Build history of the part. All positions in model axes, mm. Coordinates: 2 decimals unless noted, no trailing zeros. Order: outer loops, then holes, each group sorted by start corner. A loop starts at its lowest first (then second) coordinate and runs counter-clockwise, first axis right, second up. Notation, with made-up numbers: (87.25, 60.25) - (118.25, 60.25) arc R20 cw to (118.25, 81.25) - close; hole circle Ø3 at (47, -4.75). An arc over 180 degrees is marked (long way). Answer as CSV lines item,"result". Start each with the question number.
from build123d import *

# Parameters (mm, degrees)
SKETCH_1_W          = 160
SKETCH_1_H          = 200
EXTRUDE_2_DEPTH     = 3
SKETCH_2_R          = 1
SKETCH_2_W          = 20
SKETCH_2_H          = 40
CUT_EXTRUDE_1_DEPTH = 3
SKETCH_3_R          = 0.75
CUT_EXTRUDE_2_DEPTH = 10
SKETCH_4_R          = 1.6
CUT_EXTRUDE_3_DEPTH = 10
SKETCH_5_W          = 20
SKETCH_5_H          = 1.5
CUT_EXTRUDE_4_DEPTH = 10


with BuildPart() as part:
    # 草图1 → 凸台-拉伸2 (new body)
    with BuildSketch(Plane(origin=(0, 0, 0), x_dir=(1, 0, 0), z_dir=(0, 1, 0))):
        Rectangle(SKETCH_1_W, SKETCH_1_H)
    extrude(amount=EXTRUDE_2_DEPTH)

    # 草图2 → 切除-拉伸1 (cut)
    with BuildSketch(Plane(origin=(0, 3, 0), x_dir=(1, 0, 0), z_dir=(0, 1, 0))):
        with Locations((23, -90)):
            Circle(SKETCH_2_R)
        with Locations((13, -44)):
            Circle(SKETCH_2_R)
        with Locations((-23, -90)):
            Circle(SKETCH_2_R)
        with Locations((-23, -44)):
            Circle(SKETCH_2_R)
        with Locations((-13, -44)):
            Circle(SKETCH_2_R)
        with Locations((-13, -90)):
            Circle(SKETCH_2_R)
        with Locations((13, -90)):
            Circle(SKETCH_2_R)
        with Locations((22.939303547, -44)):
            Circle(SKETCH_2_R)
        with Locations((-18, -67)):
            Rectangle(SKETCH_2_W, SKETCH_2_H)
        with Locations((18, -67)):
            Rectangle(SKETCH_2_W, SKETCH_2_H)
    extrude(amount=-CUT_EXTRUDE_1_DEPTH, mode=Mode.SUBTRACT)

    # 草图3 → 切除-拉伸2 (cut)
    with BuildSketch(Plane(origin=(0, 3, 0), x_dir=(1, 0, 0), z_dir=(0, 1, 0))):
        with Locations((35, -10)):
            Circle(SKETCH_3_R)
        with Locations((35, 6)):
            Circle(SKETCH_3_R)
        with Locations((-1, -10)):
            Circle(SKETCH_3_R)
        with Locations((-1, 6)):
            Circle(SKETCH_3_R)
    extrude(amount=-CUT_EXTRUDE_2_DEPTH, mode=Mode.SUBTRACT)

    # 草图4 → 切除-拉伸3 (cut)
    with BuildSketch(Plane(origin=(0, 3, 0), x_dir=(1, 0, 0), z_dir=(0, 1, 0))):
        with Locations((72, 1.284440395)):
            Circle(SKETCH_4_R)
        with Locations((-72, -1.368262766)):
            Circle(SKETCH_4_R)
        with Locations((72, 92)):
            Circle(SKETCH_4_R)
        with Locations((-72, 92)):
            Circle(SKETCH_4_R)
        with Locations((-72, -92)):
            Circle(SKETCH_4_R)
        with Locations((72, -92)):
            Circle(SKETCH_4_R)
        with Locations((0, -92)):
            Circle(SKETCH_4_R)
        with Locations((0, 92)):
            Circle(SKETCH_4_R)
    extrude(amount=-CUT_EXTRUDE_3_DEPTH, mode=Mode.SUBTRACT)

    # 草图5 → 切除-拉伸4 (cut)
    with BuildSketch(Plane(origin=(0, 3, 0), x_dir=(1, 0, 0), z_dir=(0, 1, 0))):
        with Locations((-30, 77.25)):
            Rectangle(SKETCH_5_W, SKETCH_5_H)
        with Locations((-30, 30.75)):
            Rectangle(SKETCH_5_W, SKETCH_5_H)
        with Locations((15.068831665, 77.25)):
            Rectangle(SKETCH_5_W, SKETCH_5_H)
        with Locations((11.85252458, 30.75)):
            Rectangle(SKETCH_5_W, SKETCH_5_H)
    extrude(amount=-CUT_EXTRUDE_4_DEPTH, mode=Mode.SUBTRACT)


solid = part.part
(1) Probe L1, parallel to X at y = 2.3, z = 44; L2, parallel to X at y = 1.7, z = 90; L3, parallel to Z at x = 16, y = 2.8. List the from-to ranges inside material, lowest first. Write a range as [from, to].
(2) Band-saw the part on B-B on z = 80. List the corners of the cut face in (x, y), plus the area to 3 significant figures.
(3) Band-saw the part on A-A on x = -34. List the corners of the cut face in (y, z).
(4) Band-saw the part on C-C on y = 2.3. State how many separate pieces and enclosed holes the cut face has, plus the area to 3 significant figures.
Filled in:
1,L1,"x = [-80, -24], [-22, -14], [-12, 12], [14, 21.94], [23.94, 80]"
1,L2,"x = [-80, -24], [-22, -14], [-12, 12], [14, 22], [24, 80]"
1,L3,"z = [-100, -78], [-76.5, -31.5], [-30, 47], [87, 100]"
2,outline,"(-80, 0) - (-28, 0) - (-28, 3) - (-80, 3) - close; (-8, 0) - (8, 0) - (8, 3) - (-8, 3) - close; (28, 0) - (80, 0) - (80, 3) - (28, 3) - close"
2,area,"360 mm^2"
3,outline,"(0, -100) - (3, -100) - (3, -78) - (0, -78) - close; (0, -76.5) - (3, -76.5) - (3, -31.5) - (0, -31.5) - close; (0, -30) - (3, -30) - (3, 100) - (0, 100) - close"
4,separate pieces,"1"
4,enclosed holes,"26"
4,area,"30,200 mm^2"
